Here's how the part is built. I have some questions about the finished solid (model axes, mm). A direction names the side the tool comes from. Give positions to 0.01 mm unless a question says otherwise; leave off trailing zeros. Loops run counter-clockwise (first coordinate to the right, second up) from the corner with the lowest first, then second, coordinate; pieces in that order, holes last. Notation, with made-up numbers: (43, 18.5) - (51, 18.5) arc R7 cw to (51, 30.5) - close; hole circle Ø9 at (85.25, 55.5). An arc over 180 degrees is marked (long way). Return JSON: item names as keys, results as strings. Group by question number.
(1) If we section it at A-A (y = 109.5): Please give me the cut outline in (x, z).
(2) For P1, Ø12, axis at x = 146.5, z = -148.5, coming from the -Y side, with a flat end and sliding along its axis, tell me the tip position at first contact or that it passes through.
(3) If we mould it in two halves opening along X, with no side actions, what happens to faces 3 (the flat face through (-3, 457.2, -3)), 4 (the flat face through (254, 238, -4)), 5 (the flat face through (4, 238, 254))? For each: released by +X, released by -X, zero draft, split by the parting line, or undercut.
(4) I need wall thicknesses on probe 1 along X at (y, z) = (358, -98); probe 2 along Y at (x, z) = (120.5, -47). Which ranges of each line are inside material? Lowest first, please. Write a range as [from, to].
(5) If we section it at B-B (x = 26): Please give me the cut outline in (y, z), then the cut area to 3 significant figures.
(6) If we section it at C-C (z = -196.5): Please give me the cut outline in (x, y).
(7) On a 3-axis mill with a long thin cutter (end or side, diameter ignored), from which of +Z, -Z, +X, -X, +Y, -Y can I reach the whole of each face in a straight line? I mean faces 1 (the flat face through (-3, 225, -228.6)), 2 (the flat face through (-20, 0, 243)). Say none if no direction works.
Autodesk Fusion 360 part; units mm, degrees
sketch "Sketch1" plane through (0, 0, 0) normal (0, 1, 0) x (1, 0, 0)
  line L0 (228.6, -228.6) -> (-228.6, -228.6)
  line L1 (-228.6, -228.6) -> (-228.6, 228.6)
  line L2 (-228.6, 228.6) -> (228.6, 228.6)
  line L3 (228.6, 228.6) -> (228.6, -228.6)
  line L4 (228.6, -228.6) -> (-228.6, 228.6) construction
  line L5 (-228.6, -228.6) -> (228.6, 228.6) construction
  dimension "d1" = 457.2
  dimension "d2" = 457.2
extrude "Extrude1" add sketch "Sketch1" along normal blind 457.2 makes body 1
copy_body "Body->Comp1" bodies 1 removing the originals makes body 2 in component "SIzing Box"
delete_body "RemoveBody1" bodies 2 in component "SIzing Box"
sketch "Sketch1 (2)" plane through (0, 0, 0) normal (0, 1, 0) x (1, 0, 0) in component "SIzing Box"
  line L0 (228.6, -228.6) -> (-228.6, -228.6)
  line L1 (-228.6, -228.6) -> (-228.6, 228.6)
  line L2 (-228.6, 228.6) -> (228.6, 228.6)
  line L3 (228.6, 228.6) -> (228.6, -228.6)
  line L4 (228.6, -228.6) -> (-228.6, 228.6) construction
  line L5 (-228.6, -228.6) -> (228.6, 228.6) construction
  line L6 (254, -254) -> (-254, -254)
  line L7 (-254, -254) -> (-254, 254)
  line L8 (-254, 254) -> (254, 254)
  line L9 (254, 254) -> (254, -254)
  dimension "d5" = 457.2
  dimension "d6" = 457.2
  dimension "d7" = -25.4
extrude "Extrude2" add sketch "Sketch1 (2)" along normal blind 25.4 from surface at 457.2 separate body contours L0 L1 L2 L3 | L6 L7 L8 L9 makes body 3 in component "SIzing Box"
extrude "Extrude1'" add sketch "Sketch1 (2)" along normal blind 457.2 bodies 3 in component "SIzing Box"
component "SIzing Box" placed x (1, 0, 0) y (0, 1, 0) z (0, 0, 1) at (0, 0, 0)
Values:
{
 "1": {"outline": "(-254, -254) - (254, -254) - (254, 254) - (-254, 254) - close; hole (-228.6, -228.6) - (228.6, -228.6) - (228.6, 228.6) - (-228.6, 228.6) - close"},
 "2": {"P1": "y = 457.2"},
 "3": {"face 3": "undercut", "face 4": "released by +X", "face 5": "zero draft"},
 "4": {"probe 1": "[-254, -228.6], [228.6, 254]", "probe 2": "[457.2, 482.6]"},
 "5": {"outline": "(0, -254) - (482.6, -254) - (482.6, 254) - (0, 254) - (0, 228.6) - (457.2, 228.6) - (457.2, -228.6) - (0, -228.6) - close", "area": "36,100 mm2"},
 "6": {"outline": "(-254, 0) - (-228.6, 0) - (-228.6, 457.2) - (228.6, 457.2) - (228.6, 0) - (254, 0) - (254, 482.6) - (-254, 482.6) - close"},
 "7": {"face 1": "-Y", "face 2": "+Z, -Z, +X, -X, -Y"}
}
